from build123d import *

# Parameters (mm, degrees)
SKETCH1_R           = 12.065
BOSS_EXTRUDE1_DEPTH = 19.812
SKETCH2_R           = 2.921
BOSS_EXTRUDE2_DEPTH = 25.4
SKETCH3_R           = 3.556
BOSS_EXTRUDE3_DEPTH = 3.81
FILLET3_R           = 2.54
SKETCH7_R           = 2.8702
CUT_EXTRUDE1_DEPTH  = 12.7
CIRPATTERN1_COUNT   = 2
CIRPATTERN1_ANGLE   = 90
FILLET4_R           = 2.54


with BuildPart() as part:
    # Sketch1 → Boss-Extrude1 (new body)
    with BuildSketch(Plane(origin=(0, 0, 0), x_dir=(1, 0, 0), z_dir=(0, 1, 0))):
        with Locations(Location((0, 0, 0), (0, 0, 270))):
            Circle(SKETCH1_R)
    extrude(amount=BOSS_EXTRUDE1_DEPTH)

    # Sketch2 → Boss-Extrude2 (add)
    with BuildSketch(Plane(origin=(0, 19.812, 0), x_dir=(1, 0, 0), z_dir=(0, 1, 0))):
        with Locations(Location((0, 0, 0), (0, 0, 270))):
            Circle(SKETCH2_R)
    extrude(amount=BOSS_EXTRUDE2_DEPTH)

    # Sketch3 → Boss-Extrude3 (add)
    with BuildSketch(Plane(origin=(0, 45.212, 0), x_dir=(1, 0, 0), z_dir=(0, 1, 0))):
        with Locations(Location((0, 0, 0), (0, 0, 90))):
            Circle(SKETCH3_R)
    extrude(amount=BOSS_EXTRUDE3_DEPTH)

    # Fillet3
    fillet3_edges = [part.edges().sort_by_distance(p)[0] for p in [
        (0, 49.022, 3.556),
    ]]
    fillet(fillet3_edges, radius=FILLET3_R)

    # Sketch7 → Cut-Extrude1 (cut, symmetric)
    with BuildSketch(Plane.XY):
        with Locations(Location((0, 7.62, 0), (0, 0, 90.000000025))):
            Circle(SKETCH7_R)
    cut_extrude1 = extrude(amount=CUT_EXTRUDE1_DEPTH, both=True, mode=Mode.SUBTRACT)

    # CirPattern1: Cut-Extrude1 ×2 about axis
    cirpattern1_axis = Axis((0, 45.212, 0), (0, -1, 0))
    for i in range(1, CIRPATTERN1_COUNT):
        add(cut_extrude1.rotate(cirpattern1_axis, i * CIRPATTERN1_ANGLE / (CIRPATTERN1_COUNT - 1)), mode=Mode.SUBTRACT)

    # Loft1: read off the stored shape, not the designer's step
    # Loft1: loft between two sections, ruled curve by curve
    loft1_from = [
        Edge.make_bspline([(3.555943144, 45.212, 0.020108599), (3.515725946, 45.212, 7.131994887), (-3.596160342, 45.212, 7.091777689), (-3.555943144, 45.212, -0.020108599), (-3.515725946, 45.212, -7.131994887), (3.596160342, 45.212, -7.091777689), (3.555943144, 45.212, 0.020108599)], [0, 0, 0, 0, 0.5, 0.5, 0.5, 1, 1, 1, 1], 3, [1, 0.333333333, 0.333333333, 1, 0.333333333, 0.333333333, 1]),
    ]
    loft1_to = [
        Edge.make_bspline([(2.781979214, 42.672, 0.890411509), (1.001156196, 42.672, 6.454369936), (-4.562802231, 42.672, 4.673546919), (-2.781979214, 42.672, -0.890411509), (-1.001156196, 42.672, -6.454369936), (4.562802231, 42.672, -4.673546919), (2.781979214, 42.672, 0.890411509)], [0, 0, 0, 0, 0.5, 0.5, 0.5, 1, 1, 1, 1], 3, [1, 0.333333333, 0.333333333, 1, 0.333333333, 0.333333333, 1]),
    ]
    loft1 = Solid(Shell([*[Face.make_surface_from_curves(loft1_from[k], loft1_to[k]) for k in range(1)], Face(Wire(loft1_from)), Face(Wire(loft1_to))]))
    add(loft1)

    # Fillet4
    fillet4_edges = [part.edges().sort_by_distance(p)[0] for p in [
        (-2.521571155, 45.212, 2.507352171),
    ]]
    fillet(fillet4_edges, radius=FILLET4_R)


solid = part.part
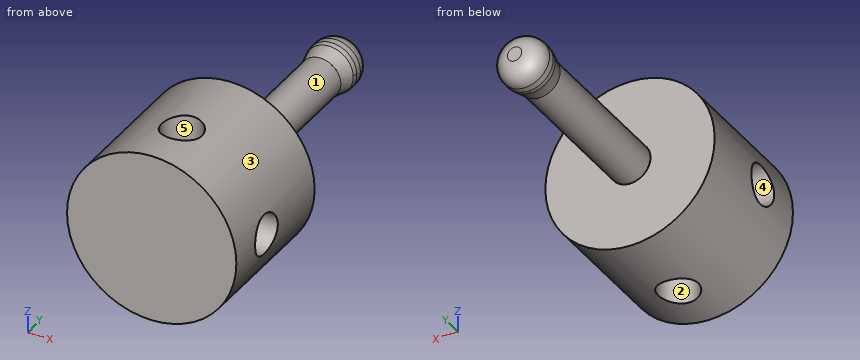
For this review, take the finished solid that the model builds, in its own axes (mm). Face numbers are marked on the shaded views. A direction names the side the tool comes from. Give positions to 0.01 mm unless a question says otherwise; leave off trailing zeros. Loops run counter-clockwise (first coordinate to the right, second up) from the corner with the lowest first, then second, coordinate; pieces in that order, holes last. Notation, with made-up numbers: (-14, 36) -> (28, 36) arc R24 cw to (28, 66) -> close; hole circle Ø6 at (17.25, 25). An arc over 180 degrees is marked (long way). One line per question, with ' | ' between items.
1) We need section D-D (y = 39). Write out the cut boundary in (x, z).
Resolved:
outline: circle Ø5.84 at (0, 0)
2) We need section B-B (y = 7.62). Write out the cut boundary in (x, z) (3 decimals), plus the area to 3 significant figures.
Resolved:
outline: (-11.719, -2.87) arc R12.065 ccw to (-2.87, -11.719) -> (-2.87, -2.87) -> close; (-11.719, 2.87) -> (-2.87, 2.87) -> (-2.87, 11.719) arc R12.065 ccw to start; (2.87, -11.719) arc R12.065 ccw to (11.719, -2.87) -> (2.87, -2.87) -> close; (2.87, 2.87) -> (11.719, 2.87) arc R12.065 ccw to (2.87, 11.719) -> close | area: 216 mm2
3) Insertion check: pin 1 Ø5 at (x, y) = (7, 16) entering from +Z; pin 2 Ø10 at (x, y) = (5, 43) entering from -Z; pin 3 Ø8 at (x, z) = (-7.5, -2.5) entering from +Y. Each pin has a flat end and moves straight along its axis. Give the tip position at first contact, or say it passes through.
Resolved:
pin 1: stops at z = 11.19 | pin 2: stops at z = -3.5 | pin 3: stops at y = 19.81
4) The part is to be moulded in two halves that separate along Z. For the marked faces 3, 4 and 5, say which applies: +Z half, -Z half, draft (parallel to the pull), parting line (faces both ways), or undercut.
Resolved:
face 3: parting line | face 4: undercut | face 5: draft
5) For the marked faces 1 and 2, list the 3-axis set-ups (+Z, -Z, +X, -X, +Y, -Y) from which the entire face can be reached by the end or side of a thin tool; tool diameter is ignored.
Resolved:
face 1: none | face 2: +Z, -Z
6) We need section A-A (x = 9). Write out the cut boundary in (y, z), plus the area to 3 significant figures.
Resolved:
outline: (0, -8.04) -> (19.81, -8.04) -> (19.81, 8.04) -> (0, 8.04) -> close; hole circle Ø5.74 at (7.62, 0) | area: 293 mm2
7) To check wall thickness, follow probe 1 along Y at (x, z) = (8, 0); probe 2 along Z at (x, y) = (5.25, 9.5); probe 3 along Y at (x, z) = (7.75, 5.5). State the ranges of each line that lie inside material, in increasing order.
Resolved:
probe 1: y = 0 to 4.75, 10.49 to 19.81 | probe 2: z = -10.86 to -2.17, 2.17 to 10.86 | probe 3: y = 0 to 19.81
8) We need section C-C (z = 7.5). Write out the cut boundary in (x, y), plus the area to 3 significant figures.
Resolved:
outline: (-9.45, 0) -> (9.45, 0) -> (9.45, 19.81) -> (-9.45, 19.81) -> close; hole circle Ø5.74 at (0, 7.62) | area: 349 mm2
